Geometry check sheet. Reference: drawing and pictorial views, mm from the part's lowest x, y, z. Round coordinates to 2 decimals unless told otherwise and drop trailing zeros. Loops run counter-clockwise (first coordinate to the right, second up) from the corner with the lowest first, then second, coordinate; pieces in that order, holes last. Notation, with made-up numbers: M 82.25,-6.75 L 107.25,-6.75 A21 cw 107.25,-0.75 Z; hole C -6,12 d7. An arc over 180 degrees is marked long. One line per question, with ' | ' between items. Start each with the question number.
(1) Draft check along X on the marked faces 1, 2 and 3. Enter one of: +X half, -X half, draft (parallel to the pull), parting line (faces both ways), or undercut.
(2) Section check A-A (x = 2.4). Record the boundary of the cut face in (y, z).
(3) Section check D-D (x = 0.3). Record the boundary of the cut face in (y, z) (1 decimal), and give its area (3 significant figures).
(4) Go/stop test with flat-tipped pins: P1, Ø1, axis at y = 2, z = 1.5, coming from the +X side; P2, Ø1, axis at x = 2, y = 2.5, coming from the -Z side. Record where each tip stops, or that it passes through.
(5) Thickness scan on probe 1 along Y at (x, z) = (1.8, 4) (1 decimal); probe 2 along Y at (x, z) = (1.7, 4.25) (1 decimal); probe 3 along X at (y, z) = (1.05, 9) (1 decimal). Record the ranges inside material, lowest first. Write a range as [from, to].
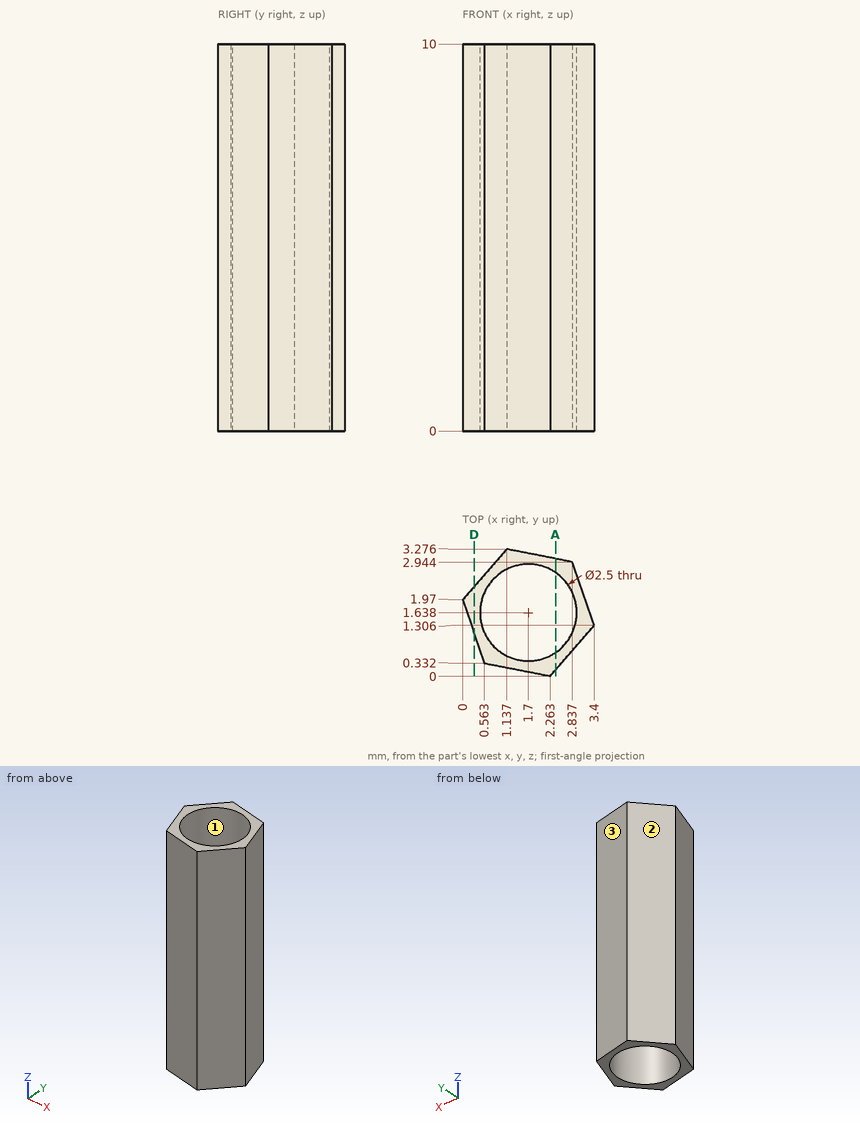
The answers:
1) face 1: undercut | face 2: -X half | face 3: +X half
2) outline: M 0.16,0 L 0.6,0 L 0.6,10 L 0.16,10 Z; M 2.67,0 L 3.03,0 L 3.03,10 L 2.67,10 Z
3) outline: M 1.1,0 L 2.3,0 L 2.3,10 L 1.1,10 Z | area: 12.2 mm²
4) P1: x = 3.33 | P2: z = 0
5) probe 1: [0.1, 0.4], [2.9, 3.1] | probe 2: [0.1, 0.4], [2.9, 3.2] | probe 3: [0.3, 0.6], [2.8, 3.2]
